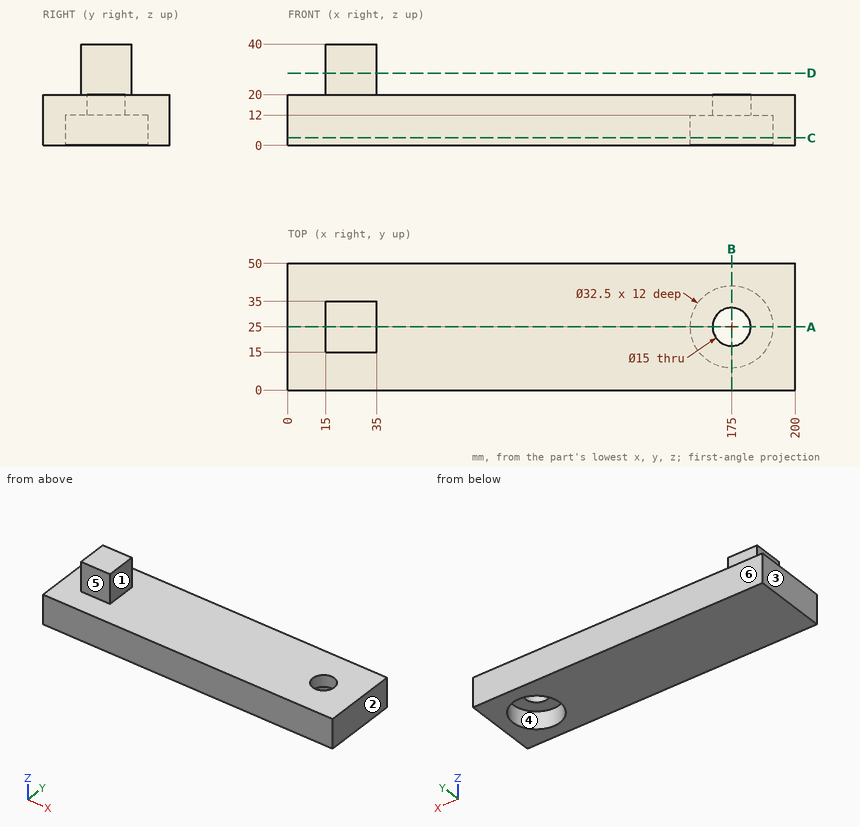
Here's the drawing with two shaded views (mm, measured from the low corner). I have some questions. A direction names the side the tool comes from. Round coordinates to 2 decimals unless told otherwise and drop trailing zeros. Order: outer loops, then holes, each group sorted by start corner. A loop starts at its lowest first (then second) coordinate and runs counter-clockwise, first axis right, second up. Notation, with made-up numbers: (53.5, 19.25) -> (69.5, 19.25) arc R35 ccw to (69.5, 51.25) -> close; hole circle Ø8 at (66.25, 2.25). An arc over 180 degrees is marked (long way). Return JSON: item names as keys, results as strings.
Q1. If we section it at B-B on x = 175: List the corners of the cut face in (y, z) for me.
Filled sheet:
{"outline": "(0, 0) -> (8.75, 0) -> (8.75, 12) -> (17.5, 12) -> (17.5, 20) -> (0, 20) -> close; (32.5, 12) -> (41.25, 12) -> (41.25, 0) -> (50, 0) -> (50, 20) -> (32.5, 20) -> close"}
Q2. If we section it at D-D on z = 28.5: List the corners of the cut face in (x, y) for me, plus the area to 3 significant figures.
Filled sheet:
{"outline": "(15, 15) -> (35, 15) -> (35, 35) -> (15, 35) -> close", "area": "400 mm^2"}
Q3. Which directions (+Z, -Z, +X, -X, +Y, -Y) give clear straight access to the entire face, cutting with the end or side of a thin tool? Please do the marked faces 1 and 2.
Filled sheet:
{"face 1": "+Z, +X, +Y, -Y", "face 2": "+Z, -Z, +X, +Y, -Y"}
Q4. I need wall thicknesses on line 1 along Y through (x, z) = (175, 4.5); line 2 along Y through (x, z) = (175, 16); line 3 along Z through (x, y) = (115, 43). Which ranges of each line are inside material? Lowest first, please. Write a range as from..to.
Filled sheet:
{"line 1": "y = 0..8.75, 41.25..50", "line 2": "y = 0..17.5, 32.5..50", "line 3": "z = 0..20"}
Q5. If we section it at A-A on y = 25: List the corners of the cut face in (x, z) for me.
Filled sheet:
{"outline": "(0, 0) -> (158.75, 0) -> (158.75, 12) -> (167.5, 12) -> (167.5, 20) -> (35, 20) -> (35, 40) -> (15, 40) -> (15, 20) -> (0, 20) -> close; (182.5, 12) -> (191.25, 12) -> (191.25, 0) -> (200, 0) -> (200, 20) -> (182.5, 20) -> close"}
Q6. If we mould it in two halves opening along Y, with no side actions, what happens to the marked faces 3, 4, 5 and 6? For each: released by +Y, released by -Y, zero draft, split by the parting line, or undercut.
Filled sheet:
{"face 3": "zero draft", "face 4": "undercut", "face 5": "released by -Y", "face 6": "released by +Y"}
Q7. For pin 1 Ø3 at (x, y) = (73, 10.5) entering from +Z; pin 2 Ø16 at (x, z) = (22.5, 31.5) entering from -Y; pin 3 Ø22 at (y, z) = (28, 33.5) entering from +X, each with a flat end and sliding along its axis, tell me the tip position at first contact or that it passes through.
Filled sheet:
{"pin 1": "stops at z = 20", "pin 2": "stops at y = 15", "pin 3": "stops at x = 35"}
Q8. If we section it at C-C on z = 3: List the corners of the cut face in (x, y) for me, plus the area to 3 significant figures.
Filled sheet:
{"outline": "(0, 0) -> (200, 0) -> (200, 50) -> (0, 50) -> close; hole circle Ø32.5 at (175, 25)", "area": "9,170 mm^2"}
